Can you work these out from the drawing? Everything is in mm from the part's minimum corner. A direction names the side the tool comes from. Round coordinates to 2 decimals unless told otherwise and drop trailing zeros. Order: outer loops, then holes, each group sorted by start corner. A loop starts at its lowest first (then second) coordinate and runs counter-clockwise, first axis right, second up. Notation, with made-up numbers: (43, 80.5) - (64, 80.5) arc R18 ccw to (64, 109.5) - close; hole circle Ø10 at (13.25, 79). An arc over 180 degrees is marked (long way). Write item = value, one per line.
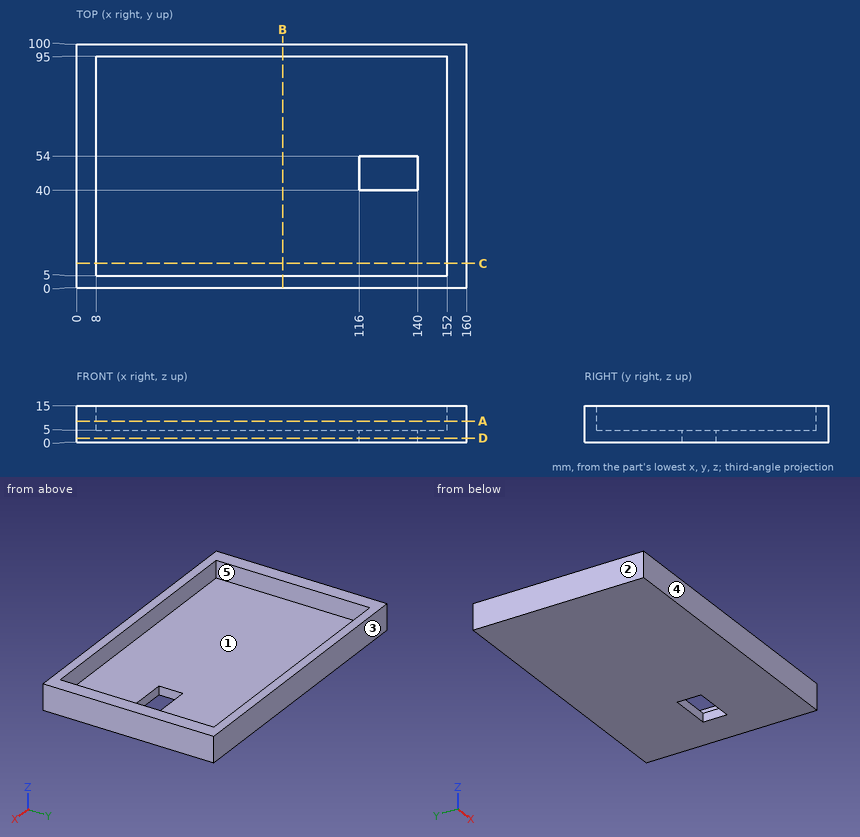
(1) On a 3-axis mill with a long thin cutter (end or side, diameter ignored), from which of +Z, -Z, +X, -X, +Y, -Y can I reach the whole of each face in a straight line? I mean the marked faces 1 and 2. Say none if no direction works.
Computed:
face_1 = +Z
face_2 = +Z, -Z, -X, +Y, -Y
(2) If we section it at A-A (z = 8.75): Write out the boundary of the cut face in (x, y), plus the area to 3 significant figures.
Computed:
outline = (0, 0) - (160, 0) - (160, 100) - (0, 100) - close; hole (8, 5) - (152, 5) - (152, 95) - (8, 95) - close
area = 3,040 mm^2
(3) If we section it at C-C (y = 10): Write out the boundary of the cut face in (x, z).
Computed:
outline = (0, 0) - (160, 0) - (160, 15) - (152, 15) - (152, 5) - (8, 5) - (8, 15) - (0, 15) - close
(4) If we section it at B-B (x = 84.5): Write out the boundary of the cut face in (y, z).
Computed:
outline = (0, 0) - (100, 0) - (100, 15) - (95, 15) - (95, 5) - (5, 5) - (5, 15) - (0, 15) - close
(5) Will these pins go through, and if not, where does the flat tip stop? P1, Ø4, axis at x = 86, z = 1.5, coming from the -Y side; P2, Ø10, axis at x = 68, y = 27.5, coming from the +Z side.
Computed:
P1 = 0
P2 = 5
(6) If I drill on line 1 (Y direction, x = 103.5, z = 11.75); line 2 (X direction, y = 44.5, z = 5.25); line 3 (Y direction, x = 133, z = 4), over which ranges is the centre line in solid material (lowest first)? Write a range as from..to.
Computed:
line_1 = 0..5, 95..100
line_2 = 0..8, 152..160
line_3 = 0..40, 54..100
(7) If we section it at D-D (z = 1.75): Write out the boundary of the cut face in (x, y), plus the area to 3 significant figures.
Computed:
outline = (0, 0) - (160, 0) - (160, 100) - (0, 100) - close; hole (116, 40) - (140, 40) - (140, 54) - (116, 54) - close
area = 15,700 mm^2
(8) Thinking about a two-plate mould opening in Y: for the marked faces 3, 4 and 5, which applies, +Y half, -Y half, draft (parallel to the pull), parting line (faces both ways), or undercut?
Computed:
face_3 = +Y half
face_4 = -Y half
face_5 = undercut
